Build history of the part. All positions in model axes, mm. Face numbers are marked on the shaded views. A direction names the side the tool comes from. Give positions to 0.01 mm unless a question says otherwise; leave off trailing zeros. Write each loop counter-clockwise with the first axis right and the second up, starting at its lowest first coordinate (ties: lowest second). Pieces come first, ordered by that corner, then holes. Notation, with made-up numbers: (39.25, -19) -> (97.25, -19) arc R24 ccw to (97.25, -6) -> close; hole circle Ø1 at (25.5, 37). An arc over 180 degrees is marked (long way). Write item = value, one per line. Start each with the question number.
Q1. Mould opens along X. For the marked faces 5, 6 and 7 say: pulls with the +X half, pulls with the -X half, needs draft (parallel to the pull), parting line crosses it, or undercut.
Q2. Saw through at C-C, the plane z = 0. List the corners of the cut face in (x, y), then the cut area to 3 significant figures.
Q3. Saw through at B-B, the plane y = 14. List the corners of the cut face in (x, z), then the cut area to 3 significant figures.
Q4. Wall check: line 1 (Z direction, x = -17, y = 18.5); line 2 (X direction, y = 13, z = -7). Give the ranges that are in metal, low to high.
Q5. Saw through at A-A, the plane x = 13. List the corners of the cut face in (y, z), then the cut area to 3 significant figures.
Q6. Saw through at D-D, the plane y = 19.5. List the corners of the cut face in (x, z), then the cut area to 3 significant figures.
Q7. Tool access for the marked faces 1, 2, 3 and 4: list every direction of +Z, -Z, +X, -X, +Y, -Y with a clear straight run to the whole face (end or side of a thin tool).
Q8. Drop flat-ended pins along their axis: P1, Ø3, axis at x = 15.5, z = -16.5, coming from the +Y side; P2, Ø12, axis at y = 12.5, z = 5, coming from the -X side; P3, Ø2, axis at x = 16.09, z = -16.09, coming from the +Y side; P4, Ø8, axis at y = 32.5, z = -9, coming from the +X side. Give the stop position or say it passes through.
from build123d import *

# Parameters (mm, degrees)
IZIM1_W                     = 42
IZIM1_H                     = 42
Y_KSEKLIK_EKSTR_ZYON1_DEPTH = 23
IZIM2_W                     = 71.608863679
IZIM2_H                     = 14.84454832
KES_EKSTR_ZYON1_DEPTH       = 0.5
PAH1_SIZE                   = 5
PAH2_SIZE                   = 5
PAH3_SIZE                   = 5
PAH4_SIZE                   = 5
IZIM3_W                     = 11.40471201
IZIM3_H                     = 14.84454832
KES_EKSTR_ZYON2_DEPTH       = 10.5
IZIM6_W                     = 48.50384319
IZIM6_H                     = 14.84454832
KES_EKSTR_ZYON3_DEPTH       = 0.5
IZIM7_W                     = 38.182763894
IZIM7_H                     = 14.84454832
KES_EKSTR_ZYON4_DEPTH       = 0.5
AYNALAMA3_COPY_1_SKETCH_W   = 11.40471201
AYNALAMA3_COPY_1_SKETCH_H   = 14.84454832
AYNALAMA3_COPY_1_DEPTH      = 10.5
AYNALAMA3_COPY_2_SKETCH_W   = 11.40471201
AYNALAMA3_COPY_2_SKETCH_H   = 14.84454832
AYNALAMA3_COPY_2_DEPTH      = 10.5
IZIM8_R                     = 1.399371897
KES_EKSTR_ZYON5_DEPTH       = 5
IZIM9_R                     = 10
Y_KSEKLIK_EKSTR_ZYON2_DEPTH = 2
KES_EKSTR_ZYON6_DEPTH       = 5
KES_EKSTR_ZYON6_DEPTH_BACK  = 2.5
IZIM10_R                    = 3.25
IZIM11_R                    = 2.5
Y_KSEKLIK_EKSTR_ZYON3_DEPTH = 20
RADYUS2_R                   = 0.5


with BuildPart() as part:
    # Çizim1 → Yükseklik-Ekstrüzyon1 (new body)
    with BuildSketch(Plane(origin=(0, 0, 0), x_dir=(1, 0, 0), z_dir=(0, 1, 0))):
        Rectangle(IZIM1_W, IZIM1_H)
    extrude(amount=Y_KSEKLIK_EKSTR_ZYON1_DEPTH)

    # Çizim2 → Kes-Ekstrüzyon1 (cut)
    with BuildSketch(Plane.XY.offset(21)):
        with Locations((-0.989717409, 11.5)):
            Rectangle(IZIM2_W, IZIM2_H)
    kes_ekstr_zyon1 = extrude(amount=-KES_EKSTR_ZYON1_DEPTH, mode=Mode.SUBTRACT)

    # Pah1
    # the kernel refuses this chamfer: 5 mm, written as the material it takes off along each edge
    with BuildSketch(Plane(origin=(-21, -12.85841494, 21), x_dir=(0.9996219169112968, 0, 0.027495876610586317), z_dir=(0, 1, 0))) as pah1_piece_1:
        Polygon((PAH1_SIZE * 0.999621916911, PAH1_SIZE * 0.0274958766106), (-PAH1_SIZE * 0.0274958766106, PAH1_SIZE * 0.999621916911), (0, 0), align=None)
    extrude(amount=29.79455572, mode=Mode.SUBTRACT)
    with BuildSketch(Plane(origin=(-21, 6.06385922, 21), x_dir=(-0.027495876610586317, 0, -0.9996219169112968), z_dir=(0, 1, 0))) as pah1_piece_2:
        Polygon((PAH1_SIZE * 0.999621916911, -PAH1_SIZE * 0.0274958766106), (-PAH1_SIZE * 0.0274958766106, -PAH1_SIZE * 0.999621916911), (0, 0), align=None)
    extrude(amount=29.79455572, mode=Mode.SUBTRACT)

    # Pah2
    # the kernel refuses this chamfer: 5 mm, written as the material it takes off along each edge
    with BuildSketch(Plane(origin=(21, -12.85841494, 21), x_dir=(-0.9996219169112968, 0, 0.027495876610586317), z_dir=(0, 1, 0)), Plane(origin=(21, 6.06385922, 21), x_dir=(-0.9996219169112968, 0, 0.027495876610586317), z_dir=(0, 1, 0))) as pah2_piece_1:
        Polygon((PAH2_SIZE * 0.999621916911, -PAH2_SIZE * 0.0274958766106), (-PAH2_SIZE * 0.0274958766106, -PAH2_SIZE * 0.999621916911), (0, 0), align=None)
    extrude(amount=29.79455572, mode=Mode.SUBTRACT)

    # Pah3
    pah3_edges = [part.edges().sort_by_distance(p)[0] for p in [
        (21, 11.5, -21),
    ]]
    chamfer(pah3_edges, length=PAH3_SIZE)

    # Pah4
    pah4_edges = [part.edges().sort_by_distance(p)[0] for p in [
        (-21, 11.5, -21),
    ]]
    chamfer(pah4_edges, length=PAH4_SIZE)

    # Çizim3 → Kes-Ekstrüzyon2 (cut)
    with BuildSketch(Plane(origin=(-25.571067812, 0, 25.571067812), x_dir=(0.707106781186546, 0, 0.707106781186549), z_dir=(-0.707106781186549, 0, 0.707106781186546))):
        with Locations((0, 11.5)):
            Rectangle(IZIM3_W, IZIM3_H)
    kes_ekstr_zyon2 = extrude(amount=-KES_EKSTR_ZYON2_DEPTH, mode=Mode.SUBTRACT)

    # Aynalama1: Kes-Ekstrüzyon1, Kes-Ekstrüzyon2 across plane
    add(kes_ekstr_zyon1.mirror(Plane.XY), mode=Mode.SUBTRACT)
    add(kes_ekstr_zyon2.mirror(Plane.XY), mode=Mode.SUBTRACT)

    # Aynalama2: Kes-Ekstrüzyon2 across plane
    add(kes_ekstr_zyon2.mirror(Plane(origin=(0, 0, 0), x_dir=(0, 0, 1), z_dir=(1, 0, 0))), mode=Mode.SUBTRACT)

    # Çizim6 → Kes-Ekstrüzyon3 (cut)
    with BuildSketch(Plane(origin=(21, 0, 0), x_dir=(0, 0, -1), z_dir=(1, 0, 0))):
        with Locations((0, 11.5)):
            Rectangle(IZIM6_W, IZIM6_H)
    extrude(amount=-KES_EKSTR_ZYON3_DEPTH, mode=Mode.SUBTRACT)

    # Çizim7 → Kes-Ekstrüzyon4 (cut)
    with BuildSketch(Plane.ZY.offset(21)):
        with Locations((0, 11.5)):
            Rectangle(IZIM7_W, IZIM7_H)
    extrude(amount=-KES_EKSTR_ZYON4_DEPTH, mode=Mode.SUBTRACT)

    # Aynalama3 copy 1 sketch → Aynalama3 copy 1 (cut)
    with BuildSketch(Plane(origin=(25.571067812, 0, -25.571067812), x_dir=(-0.707106781186546, 0, -0.707106781186549), z_dir=(0.707106781186549, 0, -0.707106781186546))):
        with Locations((0, 11.5)):
            Rectangle(AYNALAMA3_COPY_1_SKETCH_W, AYNALAMA3_COPY_1_SKETCH_H)
    extrude(amount=-AYNALAMA3_COPY_1_DEPTH, mode=Mode.SUBTRACT)

    # Aynalama3 copy 2 sketch → Aynalama3 copy 2 (cut)
    with BuildSketch(Plane(origin=(-25.571067812, 0, -25.571067812), x_dir=(0.707106781186546, 0, -0.707106781186549), z_dir=(-0.707106781186549, 0, -0.707106781186546))):
        with Locations((0, -11.5)):
            Rectangle(AYNALAMA3_COPY_2_SKETCH_W, AYNALAMA3_COPY_2_SKETCH_H)
    extrude(amount=-AYNALAMA3_COPY_2_DEPTH, mode=Mode.SUBTRACT)

    # Çizim8 → Kes-Ekstrüzyon5 (cut)
    with BuildSketch(Plane(origin=(0, 23, 0), x_dir=(1, 0, 0), z_dir=(0, 1, 0))):
        with Locations(Location((-16.087568017, 16.087568017, 0), (0, 0, 270))):
            Circle(IZIM8_R)
        with Locations(Location((16.087568017, 16.087568017, 0), (0, 0, 90))):
            Circle(IZIM8_R)
        with Locations(Location((16.087568017, -16.087568017, 0), (0, 0, 270))):
            Circle(IZIM8_R)
        with Locations(Location((-16.087568017, -16.087568017, 0), (0, 0, 90))):
            Circle(IZIM8_R)
    extrude(amount=-KES_EKSTR_ZYON5_DEPTH, mode=Mode.SUBTRACT)

    # Çizim9 → Yükseklik-Ekstrüzyon2 (add)
    with BuildSketch(Plane(origin=(0, 23, 0), x_dir=(1, 0, 0), z_dir=(0, 1, 0))):
        with Locations(Location((0, 0, 0), (0, 0, 90))):
            Circle(IZIM9_R)
    extrude(amount=Y_KSEKLIK_EKSTR_ZYON2_DEPTH)

    # Çizim10 → Kes-Ekstrüzyon6 (cut, two sides: drawn at the far end of the back side and taken through both)
    with BuildSketch(Plane(origin=(0, 23, 0), x_dir=(1, 0, 0), z_dir=(0, 1, 0)).offset(-KES_EKSTR_ZYON6_DEPTH_BACK)):
        with Locations(Location((0, 0, 0), (0, 0, 270))):
            Circle(IZIM10_R)
    extrude(amount=KES_EKSTR_ZYON6_DEPTH + KES_EKSTR_ZYON6_DEPTH_BACK, mode=Mode.SUBTRACT)

    # Çizim11 → Yükseklik-Ekstrüzyon3 (add)
    with BuildSketch(Plane(origin=(0, 20.5, 0), x_dir=(1, 0, 0), z_dir=(0, 1, 0))):
        with Locations(Location((0, 0, 0), (0, 0, 270))):
            Circle(IZIM11_R)
    extrude(amount=Y_KSEKLIK_EKSTR_ZYON3_DEPTH)

    # Radyus2
    radyus2_edges = [part.edges().sort_by_distance(p)[0] for p in [
        (0, 25, 10),
    ]]
    fillet(radyus2_edges, radius=RADYUS2_R)


solid = part.part
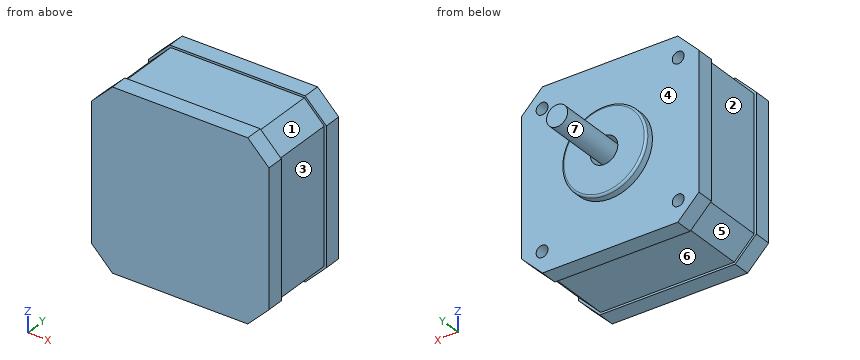
Report:
q1.face_5 = pulls with the -X half
q1.face_6 = needs draft
q1.face_7 = undercut
q2.outline = (-21, 0) -> (21, 0) -> (21, 4.08) -> (20.5, 4.08) -> (20.5, 18.92) -> (21, 18.92) -> (21, 23) -> (10, 23) -> (10, 24.5) arc R0.5 ccw to (9.5, 25) -> (3.25, 25) -> (3.25, 20.5) -> (2.5, 20.5) -> (2.5, 40.5) -> (-2.5, 40.5) -> (-2.5, 20.5) -> (-3.25, 20.5) -> (-3.25, 25) -> (-9.5, 25) arc R0.5 ccw to (-10, 24.5) -> (-10, 23) -> (-21, 23) -> (-21, 18.92) -> (-20.5, 18.92) -> (-20.5, 4.08) -> (-21, 4.08) -> close
q2.area = 1,060 mm2
q3.outline = (-20.5, -15.79) -> (-15.79, -20.5) -> (15.79, -20.5) -> (20.5, -15.79) -> (20.5, 15.79) -> (15.79, 20.5) -> (-15.79, 20.5) -> (-20.5, 15.79) -> close
q3.area = 1,640 mm2
q4.line_1 = -19.29 to -17.15, -15.03 to 15.03, 17.15 to 19.29
q4.line_2 = -20.5 to 20.5
q5.outline = (0, -21) -> (4.08, -21) -> (4.08, -20.5) -> (18.92, -20.5) -> (18.92, -21) -> (23, -21) -> (23, 21) -> (18.92, 21) -> (18.92, 20.5) -> (4.08, 20.5) -> (4.08, 21) -> (0, 21) -> close
q5.area = 951 mm2
q6.outline = (-21, -16) -> (-16, -21) -> (16, -21) -> (21, -16) -> (21, 16) -> (16, 21) -> (-16, 21) -> (-21, 16) -> close; hole circle Ø2.8 at (-16.09, -16.09); hole circle Ø2.8 at (-16.09, 16.09); hole circle Ø2.8 at (16.09, -16.09); hole circle Ø2.8 at (16.09, 16.09)
q6.area = 1,690 mm2
q7.face_1 = +Z, +X
q7.face_2 = +Z, -Z, -X
q7.face_3 = +Z, -Z, +X
q7.face_4 = +Y
q8.P1 = 23
q8.P2 = -20.5
q8.P3 = 18
q8.P4 = through
